```python
from build123d import *

# Parameters (mm, degrees)
PROFILE_LASER_PROFILE_3MM_W   = 22.6
PROFILE_LASER_PROFILE_3MM_H   = 3.1
PROFILE_LASER_PROFILE_3MM_W_2 = 15
PROFILE_LASER_PROFILE_3MM_H_2 = 19
LASER_PROFILE_3MM_DEPTH       = 3


with BuildPart() as part:
    # Profile_Laser_profile_3mm → Laser_profile_3mm (new body)
    with BuildSketch(Plane.XY):
        Polygon((0, -42.4), (2.45, -42.4), (2.45, -38.48), (5.55, -38.48), (5.55, -42.4), (30.5, -42.4), (30.5, -27), (33.5, -27), (33.5, -24), (30.5, -24), (30.5, -4), (33.5, -4), (33.5, -1), (30.5, -1), (30.5, 2), (33.5, 2), (33.5, 5), (30.5, 5), (30.5, 6.2), (0, 6.2), (0, 5), (-3, 5), (-3, 2), (0, 2), (0, -1), (-3, -1), (-3, -4), (0, -4), (0, -24), (-3, -24), (-3, -27), (0, -27), align=None)
        with Locations((15.25, -10)):
            Rectangle(PROFILE_LASER_PROFILE_3MM_W, PROFILE_LASER_PROFILE_3MM_H, mode=Mode.SUBTRACT)
        with Locations((17.5, -24.5)):
            Rectangle(PROFILE_LASER_PROFILE_3MM_W_2, PROFILE_LASER_PROFILE_3MM_H_2, mode=Mode.SUBTRACT)
    extrude(amount=LASER_PROFILE_3MM_DEPTH)


solid = part.part
```
Geometry check sheet. Reference: the model listing, model coordinates, mm. A direction names the side the tool comes from. Round coordinates to 2 decimals unless told otherwise and drop trailing zeros. Order: outer loops, then holes, each group sorted by start corner. A loop starts at its lowest first (then second) coordinate and runs counter-clockwise, first axis right, second up. Notation, with made-up numbers: (-16.75, 73) -> (16.25, 73) arc R15 cw to (16.25, 83) -> close; hole circle Ø8 at (-9.5, 48.25). An arc over 180 degrees is marked (long way). Return JSON: item names as keys, results as strings. Group by question number.
Q1. Tool access check on faces 4 (the flat face through (0, -35, 1)), 5 (the flat face through (25, -25, 1)), 6 (the flat face through (30.5, -14, 1)), 7 (the flat face through (30.5, 6, 1)). Record the directions out of +Z, -Z, +X, -X, +Y, -Y that give a thin tool (end or side, any length) a straight path to the whole face; none if there is none.
Q2. Gauge pin test, flat ends, axial feed: pin 1 (1.5 mm diameter, centred on y = -35, z = 2, fed in from +X); pin 2 (0.9 mm diameter, centred on y = -40, z = 1.5, fed in from -X); pin 3 (1.5 mm diameter, centred on x = 32, z = 1, fed in from -Y). Record the tip position at first contact, or that the pin passes through.
Q3. Section check C-C, the plane x = 4.5. Record the boundary of the cut face in (y, z), plus the area to 3 significant figures.
Q4. Section check B-B, the plane x = 16.5. Record the boundary of the cut face in (y, z), plus the area to 3 significant figures.
Q5. Section check A-A, the plane y = -17. Record the boundary of the cut face in (x, z), plus the area to 3 significant figures.
Q6. Material ranges on probe 1 along Y at (x, z) = (24, 1.55); probe 2 along X at (y, z) = (-40, 2.2); probe 3 along Y at (x, z) = (5, 0.9), recorded low to high. Write a range as from..to.
Q7. Section check D-D, the plane z = 2.25. Count the separate pieces of the cut face and the enclosed holes in it, plus the area to 3 significant figures.
Q8. Release check for a two-part mould opening along X. For faces 1 (the flat face through (-3, 4, 1)), 2 (the flat face through (-2, 2, 1)), 3 (the flat face through (2.45, -40, 1)) record: released by +X, released by -X, zero draft, split by the parting line, or undercut.
Numbers:
{
 "1": {"face 4": "+Z, -Z, -X, -Y", "face 5": "+Z, -Z", "face 6": "+Z, -Z, +X", "face 7": "+Z, -Z, +X, +Y"},
 "2": {"pin 1": "x = 30.5", "pin 2": "x = 0", "pin 3": "y = -27"},
 "3": {"outline": "(-38.48, 0) -> (-11.55, 0) -> (-11.55, 3) -> (-38.48, 3) -> close; (-8.45, 0) -> (6.2, 0) -> (6.2, 3) -> (-8.45, 3) -> close", "area": "125 mm^2"},
 "4": {"outline": "(-42.4, 0) -> (-34, 0) -> (-34, 3) -> (-42.4, 3) -> close; (-15, 0) -> (-11.55, 0) -> (-11.55, 3) -> (-15, 3) -> close; (-8.45, 0) -> (6.2, 0) -> (6.2, 3) -> (-8.45, 3) -> close", "area": "79.5 mm^2"},
 "5": {"outline": "(0, 0) -> (10, 0) -> (10, 3) -> (0, 3) -> close; (25, 0) -> (30.5, 0) -> (30.5, 3) -> (25, 3) -> close", "area": "46.5 mm^2"},
 "6": {"probe 1": "-42.4..-34, -15..-11.55, -8.45..6.2", "probe 2": "0..2.45, 5.55..30.5", "probe 3": "-38.48..-11.55, -8.45..6.2"},
 "7": {"separate pieces": "1", "enclosed holes": "2", "area": "1,170 mm^2"},
 "8": {"face 1": "released by -X", "face 2": "zero draft", "face 3": "undercut"}
}
